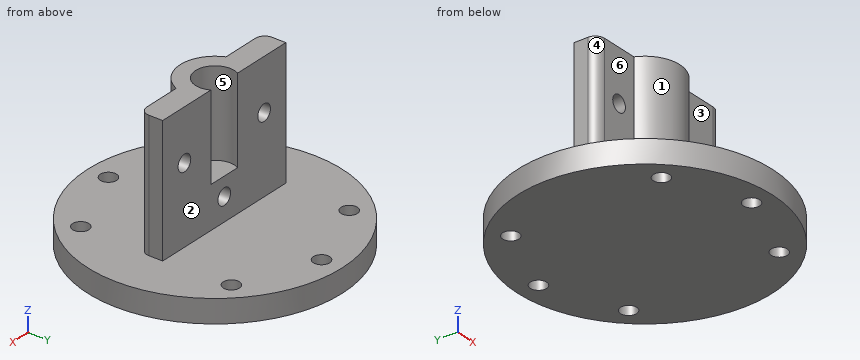
from build123d import *

# Parameters (mm, degrees)
SKETCH1_R           = 7.5
BOSS_EXTRUDE1_DEPTH = 32.5
SKETCH2_R           = 27.5
SKETCH2_R_2         = 7.5
SKETCH2_R_3         = 1.75
BOSS_EXTRUDE2_DEPTH = 5
SKETCH3_W           = 27
SKETCH3_H           = 6
CUT_EXTRUDE1_DEPTH  = 27.5
BOSS_EXTRUDE3_DEPTH = 5
BOSS_EXTRUDE4_DEPTH = 9
BOSS_EXTRUDE5_DEPTH = 27.5
SKETCH7_R           = 1.75
CUT_EXTRUDE2_DEPTH  = 52.795270054
FILLET1_R           = 2


with BuildPart() as part:
    # Sketch1 → Boss-Extrude1 (new body)
    with BuildSketch(Plane.XY):
        Circle(SKETCH1_R)
        with BuildLine():
            Line((-2.720294102, 3.2), (2.720294102, 3.2))
            ThreePointArc((2.720294102, 3.2), (0, -4.2), (-2.720294102, 3.2))
        make_face(mode=Mode.SUBTRACT)
    extrude(amount=BOSS_EXTRUDE1_DEPTH)

    # Sketch2 → Boss-Extrude2 (add)
    with BuildSketch(Plane(origin=(0, 0, 0), x_dir=(-1, 0, 0), z_dir=(0, 0, -1))):
        Circle(SKETCH2_R)
        Circle(SKETCH2_R_2, mode=Mode.SUBTRACT)
        with Locations((0, 23)):
            Circle(SKETCH2_R_3, mode=Mode.SUBTRACT)
        with Locations((16.263455967, 16.263455967)):
            Circle(SKETCH2_R_3, mode=Mode.SUBTRACT)
        with Locations((16.263455967, -16.263455967)):
            Circle(SKETCH2_R_3, mode=Mode.SUBTRACT)
        with Locations((0, -23)):
            Circle(SKETCH2_R_3, mode=Mode.SUBTRACT)
        with Locations((-16.263455967, -16.263455967)):
            Circle(SKETCH2_R_3, mode=Mode.SUBTRACT)
        with Locations((-16.263455967, 16.263455967)):
            Circle(SKETCH2_R_3, mode=Mode.SUBTRACT)
    extrude(amount=-BOSS_EXTRUDE2_DEPTH)

    # Sketch3 → Cut-Extrude1 (cut)
    with BuildSketch(Plane.XY.offset(32.5)):
        with Locations((-1.5, 5)):
            Rectangle(SKETCH3_W, SKETCH3_H)
    extrude(amount=-CUT_EXTRUDE1_DEPTH, mode=Mode.SUBTRACT)

    # Sketch4 → Boss-Extrude3 (add)
    with BuildSketch(Plane(origin=(0, 0, 0), x_dir=(-1, 0, 0), z_dir=(0, 0, -1))):
        with BuildLine():
            Line((-2.720294102, 3.2), (2.720294102, 3.2))
            ThreePointArc((2.720294102, 3.2), (0, -4.2), (-2.720294102, 3.2))
        make_face()
    extrude(amount=-BOSS_EXTRUDE3_DEPTH)

    # Sketch5 → Boss-Extrude4 (add)
    with BuildSketch(Plane.XY.offset(5)):
        with BuildLine():
            Line((-3.693237063, 2), (3.693237063, 2))
            ThreePointArc((3.693237063, 2), (0, -4.2), (-3.693237063, 2))
        make_face()
    extrude(amount=BOSS_EXTRUDE4_DEPTH)

    # Sketch6 → Boss-Extrude5 (add)
    with BuildSketch(Plane.XY.offset(5)):
        with BuildLine():
            Line((-7.228416147, 2), (-17, 2))
            Line((-17, 2), (-17, -3))
            Line((-17, -3), (-6.873863542, -3))
            ThreePointArc((-6.873863542, -3), (-7.481214682, -0.530496831), (-7.228416147, 2))
        make_face()
        with BuildLine():
            Line((6.873863542, -3), (17, -3))
            Line((17, -3), (17, 2))
            Line((17, 2), (7.228416147, 2))
            ThreePointArc((7.228416147, 2), (7.481214682, -0.530496831), (6.873863542, -3))
        make_face()
    extrude(amount=BOSS_EXTRUDE5_DEPTH)

    # Sketch7 → Cut-Extrude2 (cut, through all)
    with BuildSketch(Plane(origin=(0, 2, 0), x_dir=(1, 0, 0), z_dir=(0, 1, 0))):
        with Locations(Location((0, -10, 0), (0, 0, 270))):
            Circle(SKETCH7_R)
        with Locations(Location((-11, -21.5, 0), (0, 0, 270))):
            Circle(SKETCH7_R)
        with Locations(Location((11, -21.5, 0), (0, 0, 270))):
            Circle(SKETCH7_R)
    extrude(amount=-CUT_EXTRUDE2_DEPTH, mode=Mode.SUBTRACT)

    # Fillet1
    fillet1_edges = [part.edges().sort_by_distance(p)[0] for p in [
        (-17, -3, 18.75),
        (17, -3, 18.75),
    ]]
    fillet(fillet1_edges, radius=FILLET1_R)


solid = part.part
Source: CAD feature listing. Evaluate the final solid. Frame: model axes, mm. Face numbers are marked on the shaded views. A direction names the side the tool comes from. Coordinates: 2 decimals unless noted, no trailing zeros. Loops run counter-clockwise (first coordinate to the right, second up) from the corner with the lowest first, then second, coordinate; pieces in that order, holes last. Notation, with made-up numbers: (3.5, 40) - (23.5, 40) arc R12 cw to (23.5, 59) - close; hole circle Ø10 at (73, 63). An arc over 180 degrees is marked (long way). One line per question, with ' | ' between items.
1) Section D-D, the plane y = 23. Return loops of the section in (x, z).
Report:
outline: (-15.07, 0) - (-1.75, 0) - (-1.75, 5) - (-15.07, 5) - close; (1.75, 0) - (15.07, 0) - (15.07, 5) - (1.75, 5) - close
2) Section A-A, the plane y = 0. Return loops of the section in (x, z), then the cut area to 3 significant figures.
Report:
outline: (-27.5, 0) - (27.5, 0) - (27.5, 5) - (17, 5) - (17, 32.5) - (4.2, 32.5) - (4.2, 14) - (-4.2, 14) - (-4.2, 32.5) - (-17, 32.5) - (-17, 5) - (-27.5, 5) - close; hole circle Ø3.5 at (-11, 21.5); hole circle Ø3.5 at (0, 10); hole circle Ø3.5 at (11, 21.5) | area: 1,030 mm²
3) First-contact query: P1, Ø4, axis at x = 11, z = 21.5, coming from the +Y side; P2, Ø3, axis at x = -11, z = 21.5, coming from the +Y side; P3, Ø10, axis at y = -2.5, z = 9.5, coming from the +X side; P4, Ø5.5, axis at x = -16.26, y = 16.26, coming from the +Z side. Flat tips, straight axial feed; report the tip coordinate or a pass-through.
Report:
P1: stops at y = 2 | P2: passes through | P3: stops at x = 27.5 | P4: stops at z = 5
4) Set-up query: the marked faces 1, 2 and 3. Return all of +Z, -Z, +X, -X, +Y, -Y with unobstructed straight access to the full face (end or side cutting, diameter ignored); none if empty.
Report:
face 1: +Z, -Y | face 2: +Z, +X, -X, +Y | face 3: +Z, +X, -Y
5) Pull-direction query (X, two-part tool) for the marked faces 4, 5 and 6; classes: released by +X, released by -X, zero draft, split by the parting line, or undercut.
Report:
face 4: released by -X | face 5: undercut | face 6: zero draft
6) Section B-B, the plane x = 0. Return loops of the section in (y, z).
Report:
outline: (-27.5, 0) - (-24.75, 0) - (-24.75, 5) - (-27.5, 5) - close; (-21.25, 0) - (21.25, 0) - (21.25, 5) - (2, 5) - (2, 8.25) - (-7.5, 8.25) - (-7.5, 5) - (-21.25, 5) - close; (-7.5, 11.75) - (2, 11.75) - (2, 14) - (-4.2, 14) - (-4.2, 32.5) - (-7.5, 32.5) - close; (24.75, 0) - (27.5, 0) - (27.5, 5) - (24.75, 5) - close
7) Line query: line 1 along X through (y, z) = (16, 2); line 2 along X through (y, z) = (0, 21); line 3 along Z through (x, y) = (-23.5, 0.5). Output: solid intervals per line, ascending.
Report:
line 1: x = -22.37 to -17.99, -14.53 to 14.53, 17.99 to 22.37 | line 2: x = -17 to -12.68, -9.32 to -4.2, 4.2 to 9.32, 12.68 to 17 | line 3: z = 0 to 5
8) Section C-C, the plane x = -11. Return loops of the section in (y, z).
Report:
outline: (-25.2, 0) - (25.2, 0) - (25.2, 5) - (2, 5) - (2, 19.75) - (-3, 19.75) - (-3, 5) - (-25.2, 5) - close; (-3, 23.25) - (2, 23.25) - (2, 32.5) - (-3, 32.5) - close
